Verification items for the finished model (mm, model axes). A direction names the side the tool comes from. Give positions to 0.01 mm unless a question says otherwise; leave off trailing zeros. Write each loop counter-clockwise with the first axis right and the second up, starting at its lowest first coordinate (ties: lowest second). Pieces come first, ordered by that corner, then holes. Notation, with made-up numbers: (80, 49) -> (120, 49) arc R19 ccw to (120, 77) -> close; hole circle Ø2 at (22, 3). An arc over 180 degrees is marked (long way). Answer as CSV lines item,"result".
Autodesk Inventor part; units mm, degrees
ref_plane "YZ Plane" through (0, 0, 0) normal (1, 0, 0) x (0, 1, 0)
ref_plane "XZ Plane" through (0, 0, 0) normal (0, 1, 0) x (-1, 0, 0)
ref_plane "XY Plane" through (0, 0, 0) normal (0, 0, 1) x (1, 0, 0)
ref_plane "Work Plane1" through (0, 0, 0) normal (0, 0, 1) x (1, 0, 0)
sketch "Sketch1" plane through (0, 0, 0) normal (0, 0, 1) x (1, 0, 0)
  circle A0 centre (-15.5, 7) radius 1.45
  circle A1 centre (-15.5, -7) radius 1.45
  line L0 (63, 19) -> (63, -19)
  circle A2 centre (56, -16.5) radius 1.45
  circle A3 centre (60.5, 16.5) radius 1.45
  circle A4 centre (-15.5, 7) radius 1.45
  circle A5 centre (-15.5, -7) radius 1.45
  circle A6 centre (60.5, -16.5) radius 1.45
  circle A7 centre (56, 16.5) radius 1.45
  circle A8 centre (10, 10) radius 1.75
  circle A9 centre (-10, -10) radius 1.75
  circle A10 centre (10, -10) radius 1.75
  line L1 (31.25, -14.25) -> (31.25, 14.25)
  line L2 (31.25, 14.25) -> (59.75, 14.25)
  line L3 (59.75, 14.25) -> (59.75, -14.25)
  line L4 (59.75, -14.25) -> (31.25, -14.25)
  circle A11 centre (-10, 10) radius 1.75
  line L5 (-18, 19) -> (63, 19)
  line L6 (-18, -19) -> (-18, 19)
  line L7 (63, -19) -> (-18, -19)
  line L8 (63, 19) -> (63, -19)
  line L9 (-18, 19) -> (-13, 19)
  line L10 (-13, 19) -> (-13, -126)
  line L11 (-13, -126) -> (-18, -126)
  line L12 (-18, -126) -> (-18, 19)
  point P0 (0, 0)
  dimension "d0" = 5
  dimension "d1" = 145
extrude "Extrusion1" add sketch "Sketch1" along normal blind 8 contours L10 L7 L6 L5 | L10 L11 L12 L7
sketch "Sketch2" plane through (0, 0, 8) normal (0, 0, 1) x (1, 0, 0)
  circle A0 centre (-15.5, -7) radius 1.45
  circle A1 centre (-15.5, 7) radius 1.45
  line L0 (-13, 19) -> (-18, 19)
  line L1 (-18, 19) -> (-18, -126)
  line L2 (-18, -126) -> (-13, -126)
  line L3 (-13, -126) -> (-13, 19)
  line L4 (-18, 19) -> (-18, -126)
  line L5 (-13, -126) -> (-13, 19)
  line L6 (-18, -126) -> (-13, -126)
  line L7 (-13, -126) -> (-13, -112)
  line L8 (-13, -112) -> (-18, -112)
  line L9 (-18, -112) -> (-18, -126)
  point P0 (0, 0)
  dimension "d4" = 14
extrude "Extrusion2" add sketch "Sketch2" along normal blind 50 contours L3 L2 L1 L8
sketch "Sketch3" plane through (0, 0, 58) normal (0, 0, 1) x (1, 0, 0)
  circle A0 centre (-34.5766, 0) radius 2.4142
  line L0 (-18, -126) -> (-13, -126)
  line L1 (-13, -126) -> (-13, -112)
  line L2 (-13, -112) -> (-18, -112)
  line L3 (-18, -112) -> (-18, -126)
  line L4 (-13, 19) -> (-13, -126)
  line L5 (-18, -112) -> (-13, -112)
  line L6 (-13, -112) -> (-13, 10)
  line L7 (-13, 10) -> (-18, 10)
  line L8 (-18, 10) -> (-18, -112)
  line L9 (-18, 10) -> (-45, 10)
  line L10 (-45, 10) -> (-45, -10)
  line L11 (-45, -10) -> (-18, -10)
  line L12 (-18, -10) -> (-18, 10)
  circle A1 centre (-34.5766, 0) radius 2.5
  circle A2 centre (-34.5766, 0) radius 7.5
  point P0 (0, 0)
  dimension "d7" = 122
  dimension "d8" = 27
  dimension "d9" = 20
  dimension "d10" = 5
  dimension "d16" = 15
extrude "Extrusion3" add sketch "Sketch3" against normal blind 8 contours L3 L2 L1 L0 | L8 L7 L4 L2 | L11 L10 L9 L8
fillet "Fillet1" radius 7 8 edges at (-15.5, -112, 50) (-15.5, -112, 8) (-15.5, -126, 58) (-15.5, -126, 0) (-18, -10, 54) (-13, 10, 54) (-45, 10, 54) (-45, -10, 54)
sketch "Sketch4" plane through (-18, 19, 0) normal (-1, 0, 0) x (0, 0, 1)
  line L0 (50, -36) -> (58, -36)
  line L1 (50, -124) -> (50, -36)
  arc A0 (43, -131) -> (50, -124) centre (43, -124) ccw
  line L2 (15, -131) -> (43, -131)
  arc A1 (8, -124) -> (15, -131) centre (15, -124) ccw
  line L3 (8, 0) -> (8, -124)
  line L4 (0, 0) -> (8, 0)
  line L5 (0, -138) -> (0, 0)
  arc A2 (0, -138) -> (7, -145) centre (7, -138) ccw
  line L6 (7, -145) -> (51, -145)
  arc A3 (51, -145) -> (58, -138) centre (51, -138) ccw
  line L7 (58, -138) -> (58, -36)
  line L8 (50, -29) -> (50, -36)
  line L9 (50, -36) -> (58, -36)
  line L10 (58, -36) -> (58, -29)
  line L11 (58, -29) -> (50, -29)
  point P0 (0, -19)
extrude "Extrusion4" add sketch "Sketch4" along normal blind 2
sketch "Sketch5" plane through (-45, -3, 58) normal (-1, 0, 0) x (0, 0, 1)
  line L0 (0, 0) -> (-8, 0)
  line L1 (0, 6) -> (0, 0)
  line L2 (-8, 6) -> (0, 6)
  line L3 (-8, 0) -> (-8, 6)
  circle A0 centre (-4, 2.5827) radius 1.4
  point P0 (-58, 3)
  dimension "d17" = 2.8
extrude "Extrusion5" cut sketch "Sketch5" against normal blind 10 contours A0
pattern_circular "Circular Pattern1" count 4 over 360 about axis through (-34.5766, 0, 58) along (0, 0, -1) of "Extrusion5"
sketch "Sketch6" plane through (-13, 19, 8) normal (1, 0, 0) x (0, 0, -1)
  circle A0 centre (-46, -19.4173) radius 1.4
  point P0 (8, -19)
  point P1 (-46, -20.8173)
hole "Hole1" at (-13, -0.4173, 54) direction (-1, 0, 0) diameter 2.8 end through all counterbore diameter 7 counterbore depth 8
properties part number "06_Fluorescence_Arm"
1) Section check D-D (z = 39.5). Record the boundary of the cut face in (x, y).
Reported:
outline,"(-20, -126) -> (-13, -126) -> (-13, -112) -> (-20, -112) -> close"
2) Section check C-C (x = -30.5). Record the boundary of the cut face in (y, z).
Reported:
outline,"(-10, 50) -> (-6.3, 50) -> (-6.3, 58) -> (-10, 58) -> close; (6.3, 50) -> (10, 50) -> (10, 58) -> (6.3, 58) -> close"
3) Depth check by flat-ended pin: pin 1 (2.5 mm diameter, centred on x = -15.5, y = 7, fed in from -Z); pin 2 (4 mm diameter, centred on y = -0.42, z = 54, fed in from +X); pin 3 (5.5 mm diameter, centred on x = -17, z = 22.5, fed in from +Y). Enter the tip coordinate at first touch or a pass-through.
Reported:
pin 1,"z = 50"
pin 2,"x = -21"
pin 3,"y = -112"
4) Section check A-A (y = -29). Record the boundary of the cut face in (x, z), and give its area (3 significant figures).
Reported:
outline,"(-20, 0) -> (-13, 0) -> (-13, 8) -> (-20, 8) -> close; (-20, 50) -> (-13, 50) -> (-13, 58) -> (-20, 58) -> close"
area,"112 mm²"
5) Draft check along X on faces 4 (the cylindrical face through (-43.448, -1.659, 54.646)), 5 (the flat face through (-45, 1, 55)), 6 (the cylindrical face through (-14.161, -6.445, 3.944)). Enter one of: +X half, -X half, draft (parallel to the pull), parting line (faces both ways), or undercut.
Reported:
face 4,"draft"
face 5,"-X half"
face 6,"undercut"
6) Tool access check on faces 1 (the flat face through (-21, 0, 52)), 2 (the cylindrical face through (-16.5, -110, 47.9)), 3 (the cylindrical face through (-14.161, 7.555, 3.944)). Record the directions out of +Z, -Z, +X, -X, +Y, -Y that give a thin tool (end or side, any length) a straight path to the whole face; none if there is none.
Reported:
face 1,"+X"
face 2,"+X, -X, +Y"
face 3,"-Z"
7) Section check B-B (x = -15.5). Record the boundary of the cut face in (y, z), and give its area (3 significant figures).
Reported:
outline,"(-126, 7) arc R7 ccw to (-119, 0) -> (-8.45, 0) -> (-8.45, 8) -> (-105, 8) arc R7 cw to (-112, 15) -> (-112, 43) arc R7 cw to (-105, 50) -> (8.36, 50) -> (8.36, 58) -> (-119, 58) arc R7 ccw to (-126, 51) -> close; (-5.55, 0) -> (5.55, 0) -> (5.55, 8) -> (-5.55, 8) -> close; (8.45, 0) -> (19, 0) -> (19, 8) -> (8.45, 8) -> close; hole circle Ø7 at (-0.42, 54)"
area,"2,740 mm²"
8) Scan lines: line 1 along Y through (x, z) = (-15.5, 2.25); line 2 along X through (y, z) = (-49, 51); line 3 along Y through (x, z) = (-19, 24). Record each from-to range of solid material in increasing order.
Reported:
line 1,"-124.14 to -8.45, -5.55 to 5.55, 8.45 to 19"
line 2,"-20 to -13"
line 3,"-126 to -112"
